The drawing under review shows one solid part. Ordinate dimensions are in mm from its lowest x, y, z. A direction names the side the tool comes from. Coordinates: 2 decimals unless noted, no trailing zeros. Loops run counter-clockwise (first coordinate to the right, second up) from the corner with the lowest first, then second, coordinate; pieces in that order, holes last. Notation, with made-up numbers: (43.5, 56) - (89.5, 56) arc R21 cw to (89.5, 89) - close; hole circle Ø5 at (-29.5, 27). An arc over 180 degrees is marked (long way). Answer as a JSON object with one key per item and string values. Group by question number.
Item 1: Clearance check with flat-ended pins moving along their axes: pin 1 (2 mm diameter, centred on x = 4.1, y = 4.48, fed in from -Z); pin 2 (3.5 mm diameter, centred on x = 4, y = 2.5, fed in from +Z). State where each tip first meets the part, or that it passes through.
Item 2: We need section A-A (z = 3.75). Give the boundary of the cut face in (x, y), then the cut area to 3 significant figures.
Item 3: We need section C-C (y = 6.5). Give the boundary of the cut face in (x, z).
Item 4: To check wall thickness, follow line 1 (X direction, y = 1.75, z = 5); line 2 (Z direction, x = 4.75, y = 7.75); line 3 (X direction, y = 5.75, z = 1.25). State the ranges of each line that lie inside material, in increasing order.
Item 5: We need section D-D (y = 3.5). Give the boundary of the cut face in (x, z).
Item 6: Tool access review of the marked faces 1 and 2: name each direction out of +Z, -Z, +X, -X, +Y, -Y from which nothing blocks a thin tool from reaching the whole face with its end or side.
Item 7: We need section B-B (x = 4). Give the boundary of the cut face in (y, z) (1 decimal).
Item 8: Mouldability with a two-part tool opening along X and no side actions: class the marked faces 3, 4 and 5 as released by +X, released by -X, zero draft, split by the parting line, or undercut.
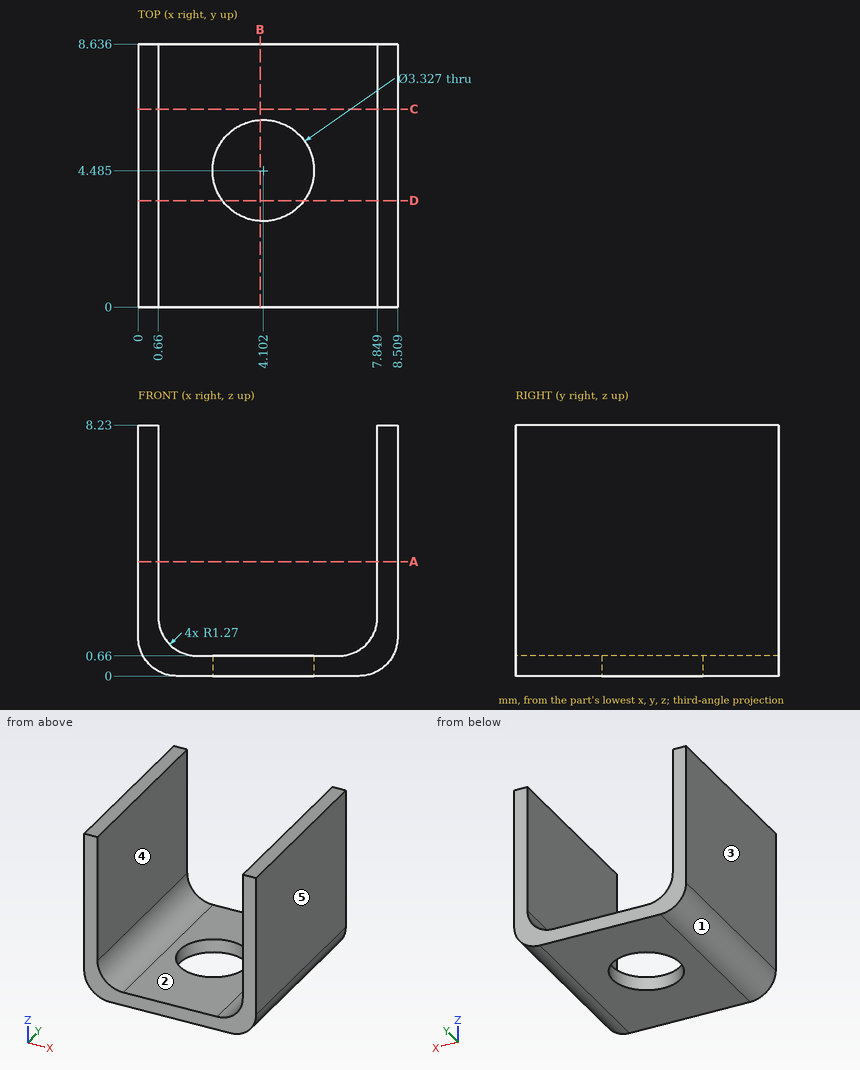
Check sheet entries:
{
 "1": {"pin 1": "passes through", "pin 2": "stops at z = 0.66"},
 "2": {"outline": "(0, 0) - (0.66, 0) - (0.66, 8.64) - (0, 8.64) - close; (7.85, 0) - (8.51, 0) - (8.51, 8.64) - (7.85, 8.64) - close", "area": "11.4 mm2"},
 "3": {"outline": "(0, 1.27) arc R1.27 ccw to (1.27, 0) - (7.24, 0) arc R1.27 ccw to (8.51, 1.27) - (8.51, 8.23) - (7.85, 8.23) - (7.85, 1.93) arc R1.27 cw to (6.58, 0.66) - (1.93, 0.66) arc R1.27 cw to (0.66, 1.93) - (0.66, 8.23) - (0, 8.23) - close"},
 "4": {"line 1": "x = 0 to 0.66, 7.85 to 8.51", "line 2": "z = 0 to 0.66", "line 3": "x = 0 to 0.86, 7.65 to 8.51"},
 "5": {"outline": "(0, 1.27) arc R1.27 ccw to (1.27, 0) - (2.76, 0) - (2.76, 0.66) - (1.93, 0.66) arc R1.27 cw to (0.66, 1.93) - (0.66, 8.23) - (0, 8.23) - close; (5.44, 0) - (7.24, 0) arc R1.27 ccw to (8.51, 1.27) - (8.51, 8.23) - (7.85, 8.23) - (7.85, 1.93) arc R1.27 cw to (6.58, 0.66) - (5.44, 0.66) - close"},
 "6": {"face 1": "-Z, -X, +Y, -Y", "face 2": "+Z, +Y, -Y"},
 "7": {"outline": "(0, 0) - (2.8, 0) - (2.8, 0.7) - (0, 0.7) - close; (6.1, 0) - (8.6, 0) - (8.6, 0.7) - (6.1, 0.7) - close"},
 "8": {"face 3": "released by -X", "face 4": "undercut", "face 5": "released by +X"}
}
